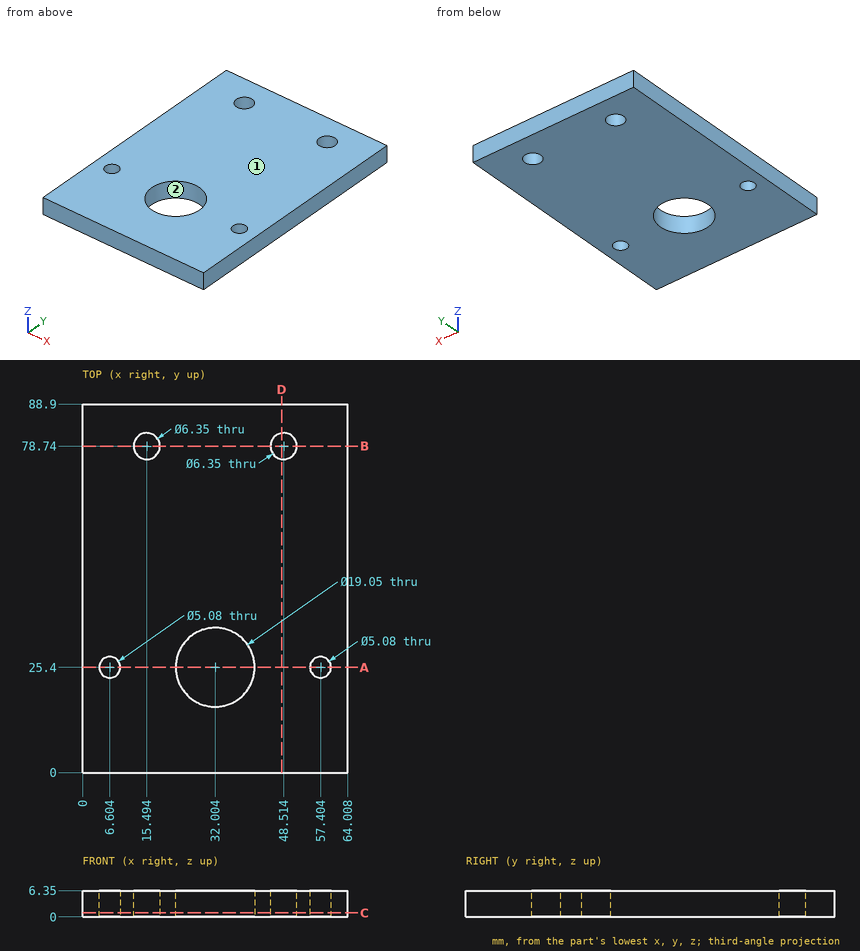
Answer from the drawing. Dimensions are ordinates in mm from the lowest x, y and z of the part. Give positions to 0.01 mm unless a question says otherwise; leave off trailing zeros. Loops run counter-clockwise (first coordinate to the right, second up) from the corner with the lowest first, then second, coordinate; pieces in that order, holes last. Notation, with made-up numbers: (78.5, 19.5) -> (86.5, 19.5) arc R16 cw to (86.5, 43.5) -> close; hole circle Ø8 at (-37, 19.25). An arc over 180 degrees is marked (long way). Use a Markdown table: item, result.
Q1. Section B-B, the plane y = 78.74 is taken. Determine the outline of the cut face in (x, z).
Solved:
| item | result |
|---|---|
| outline | (0, 0) -> (12.32, 0) -> (12.32, 6.35) -> (0, 6.35) -> close; (18.67, 0) -> (45.34, 0) -> (45.34, 6.35) -> (18.67, 6.35) -> close; (51.69, 0) -> (64.01, 0) -> (64.01, 6.35) -> (51.69, 6.35) -> close |
Q2. Find the intervals of material crossed by line 1 along Y through (x, z) = (32, 5.5) (3 decimals); line 2 along Y through (x, z) = (57, 5); line 3 along X through (y, z) = (28, 4.75), in increasing order.
Solved:
| item | result |
|---|---|
| line 1 | y = 0 to 15.875, 34.925 to 88.9 |
| line 2 | y = 0 to 22.89, 27.91 to 88.9 |
| line 3 | x = 0 to 22.84, 41.17 to 64.01 |
Q3. This flat-tipped pin is pushed along its axis until it touches: pin 1 (4 mm diameter, centred on x = 6.604, y = 25.4, fed in from -Z). Where does it stop, or does it pass through?
Solved:
| item | result |
|---|---|
| pin 1 | passes through |
Q4. Section C-C, the plane z = 1 is taken. Determine the outline of the cut face in (x, y) (3 decimals).
Solved:
| item | result |
|---|---|
| outline | (0, 0) -> (64.008, 0) -> (64.008, 88.9) -> (0, 88.9) -> close; hole circle Ø5.08 at (6.604, 25.4); hole circle Ø6.35 at (15.494, 78.74); hole circle Ø19.05 at (32.004, 25.4); hole circle Ø6.35 at (48.514, 78.74); hole circle Ø5.08 at (57.404, 25.4) |
Q5. Section A-A, the plane y = 25.4 is taken. Determine the outline of the cut face in (x, z).
Solved:
| item | result |
|---|---|
| outline | (0, 0) -> (4.06, 0) -> (4.06, 6.35) -> (0, 6.35) -> close; (9.14, 0) -> (22.48, 0) -> (22.48, 6.35) -> (9.14, 6.35) -> close; (41.53, 0) -> (54.86, 0) -> (54.86, 6.35) -> (41.53, 6.35) -> close; (59.94, 0) -> (64.01, 0) -> (64.01, 6.35) -> (59.94, 6.35) -> close |
Q6. Determine the mould class of the marked faces 1 and 2 for opening direction Y: pulls with the +Y half, pulls with the -Y half, needs draft (parallel to the pull), parting line crosses it, or undercut.
Solved:
| item | result |
|---|---|
| face 1 | needs draft |
| face 2 | undercut |
Q7. Section D-D, the plane x = 48 is taken. Determine the outline of the cut face in (y, z), then the cut area to 3 significant figures.
Solved:
| item | result |
|---|---|
| outline | (0, 0) -> (75.61, 0) -> (75.61, 6.35) -> (0, 6.35) -> close; (81.87, 0) -> (88.9, 0) -> (88.9, 6.35) -> (81.87, 6.35) -> close |
| area | 525 mm^2 |
